from build123d import *

# Parameters (mm, degrees)
BOSS_EXTRUDE1_DEPTH     = 3
SKETCH5_W               = 150
SKETCH5_H               = 20
BOSS_EXTRUDE2_DEPTH     = 3
MIRROR2_COPY_1_SKETCH_W = 150
MIRROR2_COPY_1_SKETCH_H = 20
MIRROR2_COPY_1_DEPTH    = 3
SKETCH6_W               = 23
SKETCH6_H               = 150
BOSS_EXTRUDE3_DEPTH     = 3
MIRROR4_COPY_1_SKETCH_W = 23
MIRROR4_COPY_1_SKETCH_H = 150
MIRROR4_COPY_1_DEPTH    = 3
MIRROR4_COPY_2_SKETCH_W = 23
MIRROR4_COPY_2_SKETCH_H = 150
MIRROR4_COPY_2_DEPTH    = 3
FILLET1_R               = 2
SKETCH4_W               = 35
SKETCH4_H               = 115
CUT_EXTRUDE1_DEPTH      = 10
TAP_DRILL_FOR_M3_TAP2_D = 2.5
TAP_DRILL_FOR_M3_TAP3_D = 2.5
M3_CLEARANCE_HOLE1_D    = 3.4


with BuildPart() as part:
    # Sketch1 → Boss-Extrude1 (new body)
    with BuildSketch(Plane.XY):
        Polygon((0, 195.984444731), (-138.581929877, 138.581929877), (-195.984444731, 0), (-138.581929877, -138.581929877), (0, -195.984444731), (138.581929877, -138.581929877), (195.984444731, 0), (138.581929877, 138.581929877), align=None)
    boss_extrude1 = extrude(amount=BOSS_EXTRUDE1_DEPTH)

    # Sketch5 → Boss-Extrude2 (add)
    with BuildSketch(Plane(origin=(-69.290964938, -167.283187304, 0), x_dir=(0.923879533, -0.382683432, 0), z_dir=(-0.382683432, -0.923879533, 0))):
        with Locations((0, -10)):
            Rectangle(SKETCH5_W, SKETCH5_H)
    boss_extrude2 = extrude(amount=-BOSS_EXTRUDE2_DEPTH)

    # Mirror1: Boss-Extrude2 across plane
    add(boss_extrude2.mirror(Plane.ZX))

    # Mirror2: Boss-Extrude2 across plane
    add(boss_extrude2.mirror(Plane(origin=(0, 0, 0), x_dir=(0, 0, 1), z_dir=(1, 0, 0))))

    # Mirror2 copy 1 sketch → Mirror2 copy 1 (add)
    with BuildSketch(Plane(origin=(69.290964938, 167.283187304, 0), x_dir=(-0.923879533, 0.382683432, 0), z_dir=(0.382683432, 0.923879533, 0))):
        with Locations((0, -10)):
            Rectangle(MIRROR2_COPY_1_SKETCH_W, MIRROR2_COPY_1_SKETCH_H)
    extrude(amount=-MIRROR2_COPY_1_DEPTH)

    # Sketch6 → Boss-Extrude3 (add)
    with BuildSketch(Plane(origin=(-167.283187304, -69.290964938, 0), x_dir=(0, 0, 1), z_dir=(-0.923879533, -0.382683432, 0))):
        with Locations((-8.5, 0)):
            Rectangle(SKETCH6_W, SKETCH6_H)
    boss_extrude3 = extrude(amount=-BOSS_EXTRUDE3_DEPTH)

    # Mirror3: Boss-Extrude3 across plane
    add(boss_extrude3.mirror(Plane.ZX))

    # Mirror4: Boss-Extrude1 across plane
    add(boss_extrude1.mirror(Plane(origin=(0, 0, 0), x_dir=(0, 0, 1), z_dir=(1, 0, 0))))

    # Mirror4 copy 1 sketch → Mirror4 copy 1 (add)
    with BuildSketch(Plane(origin=(167.283187304, 69.290964938, 0), x_dir=(0, 0, 1), z_dir=(0.923879533, 0.382683432, 0))):
        with Locations((-8.5, 0)):
            Rectangle(MIRROR4_COPY_1_SKETCH_W, MIRROR4_COPY_1_SKETCH_H)
    extrude(amount=-MIRROR4_COPY_1_DEPTH)

    # Mirror4 copy 2 sketch → Mirror4 copy 2 (add)
    with BuildSketch(Plane(origin=(167.283187304, -69.290964938, 0), x_dir=(0, 0, 1), z_dir=(0.923879533, -0.382683432, 0))):
        with Locations((-8.5, 0)):
            Rectangle(MIRROR4_COPY_2_SKETCH_W, MIRROR4_COPY_2_SKETCH_H)
    extrude(amount=-MIRROR4_COPY_2_DEPTH)

    # Fillet1
    fillet1_edges = [part.edges().sort_by_distance(p)[0] for p in [
        (-164.511548707, -68.142914641, 0),
        (-164.511548707, 68.142914641, 0),
        (164.511548707, 68.142914641, 0),
        (164.511548707, -68.142914641, 0),
        (-68.142914641, 164.511548707, 0),
        (68.142914641, 164.511548707, 0),
        (-68.142914641, -164.511548707, 0),
        (68.142914641, -164.511548707, 0),
    ]]
    fillet(fillet1_edges, radius=FILLET1_R)

    # Sketch4 → Cut-Extrude1 (cut)
    with BuildSketch(Plane(origin=(0, 0, 0), x_dir=(-1, 0, 0), z_dir=(0, 0, -1))):
        with Locations((-142.5, 0)):
            Rectangle(SKETCH4_W, SKETCH4_H)
        with Locations((125, 0)):
            Rectangle(SKETCH4_W, SKETCH4_H)
    extrude(amount=-CUT_EXTRUDE1_DEPTH, mode=Mode.SUBTRACT)

    # Tap Drill for M3 Tap2 (through all)
    with Locations(Plane(origin=(0, 0, 0), x_dir=(-1, 0, 0), z_dir=(0, 0, -1))):
        with Locations((-19.343368816, -169.062877249), (20.628515922, -169.078590597)):
            Hole(TAP_DRILL_FOR_M3_TAP2_D / 2)

    # Tap Drill for M3 Tap3 (through all)
    with Locations(Plane(origin=(0, 0, 0), x_dir=(-1, 0, 0), z_dir=(0, 0, -1))):
        with Locations((-20, -78.890298866), (20, -78.890298866)):
            Hole(TAP_DRILL_FOR_M3_TAP3_D / 2)

    # M3 Clearance Hole1 (through all)
    with Locations(Plane.XY.offset(3)):
        with Locations((-49.680592478, -98.01502722), (-71.876231555, -151.600040105), (-94.950689571, -79.263539034), (-117.146328648, -132.848551919)):
            Hole(M3_CLEARANCE_HOLE1_D / 2)


solid = part.part
Geometry check sheet. Reference: the model listing, model coordinates, mm. A direction names the side the tool comes from. Give positions to 0.01 mm unless a question says otherwise; leave off trailing zeros. Order: outer loops, then holes, each group sorted by start corner. A loop starts at its lowest first (then second) coordinate and runs counter-clockwise, first axis right, second up.
1) Draft check along X on faces 1 (the flat face through (-3, 3, 3)), 2 (the cylindrical face through (-66.97, -164.38, -0.6)). Enter one of: released by +X, released by -X, zero draft, split by the parting line, or undercut.
Results are:
face 1: zero draft
face 2: undercut
2) Gauge pin test, flat ends, axial feed: pin 1 (6 mm diameter, centred on x = 23.5, z = -10, fed in from +Y); pin 2 (0.9 mm diameter, centred on x = -131, z = 2, fed in from +Y); pin 3 (5 mm diameter, centred on x = 48, y = 9, fed in from -Z). Record the tip position at first contact, or that the pin passes through.
Results are:
pin 1: stops at y = 187.49
pin 2: stops at y = 141.91
pin 3: stops at z = 0
3) Cross-section at A-A (z = -13.75). Record the boundary of the cut face in (x, y), then the cut area to 3 significant figures.
Results are:
outline: (-195.98, 0) - (-138.58, -138.58) - (0, -195.98) - (138.58, -138.58) - (195.98, 0) - (138.58, 138.58) - (0, 195.98) - (-138.58, 138.58) - close; hole (-192.74, 0) - (-136.29, -136.29) - (0, -192.74) - (136.29, -136.29) - (192.74, 0) - (136.29, 136.29) - (0, 192.74) - (-136.29, 136.29) - close
area: 3,570 mm2
4) Tool access check on faces 3 (the flat face through (69.097, -164.116, -10.874)), 4 (the flat face through (-162, -77, -20)). Record the directions out of +Z, -Z, +X, -X, +Y, -Y that give a thin tool (end or side, any length) a straight path to the whole face; none if there is none.
Results are:
face 3: -Z
face 4: -Z, +X, -X, +Y, -Y
5) Cross-section at B-B (y = 14). Give the number of separate pieces and of enclosed holes in the cut face, then the cut area to 3 significant figures.
Results are:
separate pieces: 3
enclosed holes: 0
area: 1,060 mm2
6) Material ranges on probe 1 along Y at (x, z) = (20, 1); probe 2 along X at (y, z) = (-14.5, -16); probe 3 along X at (y, z) = (-70, -5.75), recorded low to high.
Results are:
probe 1: y = -187.7 to -170.13, -168 to -80.14, -77.64 to 187.7
probe 2: x = -189.98 to -186.73, 186.73 to 189.98
probe 3: x = -166.99 to -163.74, 163.74 to 166.99
